Autodesk Inventor part; units mm, degrees
ref_plane "YZ Plane" through (0, 0, 0) normal (1, 0, 0) x (0, 1, 0)
ref_plane "XZ Plane" through (0, 0, 0) normal (0, 1, 0) x (-1, 0, 0)
ref_plane "XY Plane" through (0, 0, 0) normal (0, 0, 1) x (1, 0, 0)
sketch "Sketch1" plane through (0, 0, 0) normal (0, 0, 1) x (1, 0, 0)
  circle A0 centre (0, 0) radius 25
  dimension "d0" = 50
extrude "Lens Body" add sketch "Sketch1" along normal blind 70
sketch "Sketch2" plane through (0, 0, 0) normal (0, 0, -1) x (-1, 0, 0)
  circle A0 centre (0, 0) radius 12.45
  circle A1 centre (0, 0) radius 10.95
  dimension "d3" = 24.9
  dimension "d4" = 1.5
extrude "Camera Mount" add sketch "Sketch2" along normal blind 5
sketch "Sketch4" plane through (0, 0, 0) normal (1, 0, 0) x (0, 1, 0)
  line L0 (25, 70) -> (-25, 70)
  line L1 (25, 0) -> (-25, 0)
  line L2 (25, 70) -> (-25, 70)
  line L3 (-25, 0) -> (-25, 70)
  line L4 (25, 70) -> (-25, 70)
  line L5 (-25, 70) -> (-25, 67)
  line L6 (-25, 67) -> (25, 67)
  line L7 (25, 67) -> (25, 70)
  line L8 (25, 70) -> (-25, 70)
  line L9 (23.5, 70) -> (23.5, 67)
  line L10 (0, 70) -> (0, 67)
  line L11 (-23.5, 70) -> (-23.5, 67)
  arc A0 (23.5, 67) -> (-23.5, 67) centre (0, 3.1082) ccw
  line L12 (0, -20.2369) -> (0, 86.4217)
  point P0 (0, 0)
  point P1 (12.6451, 70)
  point P2 (0, 71.1847)
  dimension "d7" = 3
  dimension "d8" = 47
revolve "Remove Material" cut sketch "Sketch4" angle 360 about axis through (0, 0, -10) along (0, 0, 1) contours L9 A0 L0
revolve "Convex Lens Shape" add sketch "Sketch4" angle 360 about axis through (0, 0, -10) along (0, 0, 1) picked at (7.0342, 70.2191) contours L0 L12 A0
shell "Hollow Out" thickness 1.5 removed faces 1 at (3.1259, -0.8227, 0)
properties part number "35mmLens"
Check sheet for the modelled part. Datum: model origin and axes. Units: mm. A direction names the side the tool comes from. Round coordinates to 2 decimals unless told otherwise and drop trailing zeros. Loops run counter-clockwise (first coordinate to the right, second up) from the corner with the lowest first, then second, coordinate; pieces in that order, holes last. Notation, with made-up numbers: M 21.25,12.25 L 57.25,12.25 A26 ccw 57.25,29.25 Z; hole C 33,-2 d5. An arc over 180 degrees is marked long. One line per question, with ' | ' between items. Start each with the question number.
Item 1: Scan lines: probe 1 along Y at (x, z) = (0, 28); probe 2 along Y at (x, z) = (0, -3); probe 3 along X at (y, z) = (16.5, 41). Record each from-to range of solid material in increasing order.
Item 2: Section check A-A (z = 46). Record the boundary of the cut face in (x, y), and give its area (3 significant figures).
Item 3: Gauge pin test, flat ends, axial feed: pin 1 Ø4 at (x, y) = (11, -17.5) entering from -Z; pin 2 Ø10 at (y, z) = (15.5, 40) entering from +X; pin 3 Ø13 at (x, y) = (0, 0) entering from -Z; pin 4 Ø25 at (x, y) = (1.5, -11) entering from +Z. Record the tip position at first contact, or that the pin passes through.
Item 4: Release check for a two-part mould opening along X. For faces 4 (the face through (10.84, 20.85, 33)), 5 (the face through (23.846, -7.509, 34.51)), 6 (the face through (-17, -17, 70)) record: released by +X, released by -X, zero draft, split by the parting line, or undercut.
Item 5: Set-up check for faces 1 (the face through (9.18, -8.41, -2.46)), 2 (the face through (7.1, 22.4, 68.5)), 3 (the face through (5, 10, 1.5)): record each of +Z, -Z, +X, -X, +Y, -Y from which the full face is reachable in a straight line by a thin tool's end or side.
Worked out:
1) probe 1: -25 to -23.5, 23.5 to 25 | probe 2: -12.45 to -10.95, 10.95 to 12.45 | probe 3: -18.78 to -16.73, 16.73 to 18.78
2) outline: C 0,0 d50; hole C 0,0 d47 | area: 229 mm^2
3) pin 1: z = 0 | pin 2: x = 22.69 | pin 3: z = 69.37 | pin 4: z = 71.18
4) face 4: undercut | face 5: split by the parting line | face 6: zero draft
5) face 1: -Z | face 2: +Z | face 3: none
